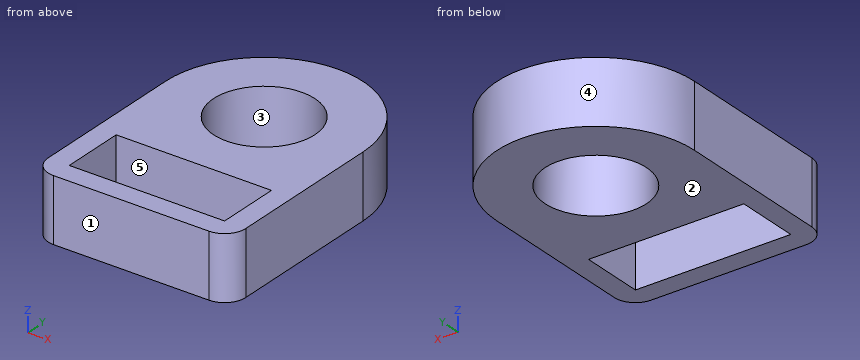
from build123d import *

# Parameters (mm, degrees)
SKETCH1_R           = 12
SKETCH1_W           = 36.78
SKETCH1_H           = 15
BOSS_EXTRUDE1_DEPTH = 15


with BuildPart() as part:
    # Sketch1 → Boss-Extrude1 (new body)
    with BuildSketch(Plane.XY):
        with BuildLine():
            Line((-18.39, -12.5), (18.390366936, -12.5))
            ThreePointArc((18.390366936, -12.5), (21.932962966, -11.028457647), (23.390326957, -7.480005346))
            Line((23.390326957, -7.480005346), (23.390326957, 30.02))
            ThreePointArc((23.390326957, 30.02), (0.000163479, 53.410163479), (-23.39, 30.02))
            Line((-23.39, 30.02), (-23.39, -7.5))
            ThreePointArc((-23.39, -7.5), (-21.925533906, -11.035533906), (-18.39, -12.5))
        make_face()
        with Locations((0, 30.02)):
            Circle(SKETCH1_R, mode=Mode.SUBTRACT)
        Rectangle(SKETCH1_W, SKETCH1_H, mode=Mode.SUBTRACT)
    extrude(amount=BOSS_EXTRUDE1_DEPTH)


solid = part.part
CAD build for the part. Positions are in the model's coordinates, mm. Face numbers are marked on the shaded views. A direction names the side the tool comes from. Coordinates: 2 decimals unless noted, no trailing zeros. Order: outer loops, then holes, each group sorted by start corner. A loop starts at its lowest first (then second) coordinate and runs counter-clockwise, first axis right, second up.
Item 1: Drill centre lines: L1, parallel to Y at x = 0, z = 9.5; L2, parallel to Y at x = -3, z = 12; L3, parallel to X at y = 30, z = 10. Where is each one in solid material? Low to high.
Check sheet entries:
L1: y = -12.5 to -7.5, 7.5 to 18.02, 42.02 to 53.41
L2: y = -12.5 to -7.5, 7.5 to 18.4, 41.64 to 53.22
L3: x = -23.39 to -12, 12 to 23.39
Item 2: Band-saw the part on B-B on x = 0. List the corners of the cut face in (y, z).
Check sheet entries:
outline: (-12.5, 0) - (-7.5, 0) - (-7.5, 15) - (-12.5, 15) - close; (7.5, 0) - (18.02, 0) - (18.02, 15) - (7.5, 15) - close; (42.02, 0) - (53.41, 0) - (53.41, 15) - (42.02, 15) - close
Item 3: Band-saw the part on D-D on x = 17.5. List the corners of the cut face in (y, z).
Check sheet entries:
outline: (-12.5, 0) - (-7.5, 0) - (-7.5, 15) - (-12.5, 15) - close; (7.5, 0) - (45.54, 0) - (45.54, 15) - (7.5, 15) - close
Item 4: Two-plate mould, pull along Y, no slides. Class the marked faces 1, 2 and 3: +Y half, -Y half, draft (parallel to the pull), parting line (faces both ways), or undercut.
Check sheet entries:
face 1: -Y half
face 2: draft
face 3: undercut
Item 5: 3-axis set-ups, long thin cutter, end or side, ignore diameter. For the marked faces 4 and 5: which of +Z, -Z, +X, -X, +Y, -Y reach the whole face in a straight line?
Check sheet entries:
face 4: +Z, -Z, +Y
face 5: +Z, -Z
Item 6: Band-saw the part on C-C on z = 8.5. List the corners of the cut face in (x, y).
Check sheet entries:
outline: (-23.39, -7.5) arc R5 ccw to (-18.39, -12.5) - (18.39, -12.5) arc R5 ccw to (23.39, -7.48) - (23.39, 30.02) arc R23.39 ccw to (-23.39, 30.02) - close; hole (-18.39, -7.5) - (18.39, -7.5) - (18.39, 7.5) - (-18.39, 7.5) - close; hole circle Ø24 at (0, 30.02)
Item 7: Band-saw the part on A-A on y = -3. List the corners of the cut face in (x, z).
Check sheet entries:
outline: (-23.39, 0) - (-18.39, 0) - (-18.39, 15) - (-23.39, 15) - close; (18.39, 0) - (23.39, 0) - (23.39, 15) - (18.39, 15) - close
Item 8: Pin check, flat tips, straight feed: pin 1 Ø2 at (y, z) = (45, 11) entering from +X; pin 2 Ø6 at (x, z) = (-14, 12) entering from +Y; pin 3 Ø14.5 at (x, y) = (0, 30.02) entering from -Z; pin 4 Ø2 at (x, z) = (9, 4) entering from +Y. Stop position of each tip, or through.
Check sheet entries:
pin 1: stops at x = 18.75
pin 2: stops at y = 50.66
pin 3: passes through
pin 4: stops at y = 52
